Design review of the part shown in the three views and the two pictorial views. Dimensions are in mm from the part's minimum x, y and z. A direction names the side the tool comes from. Round coordinates to 2 decimals unless told otherwise and drop trailing zeros. Write each loop counter-clockwise with the first axis right and the second up, starting at its lowest first coordinate (ties: lowest second). Pieces come first, ordered by that corner, then holes. Notation, with made-up numbers: (-16, 36.25) -> (28, 36.25) arc R18 ccw to (28, 47.25) -> close; hole circle Ø5 at (88.5, 50.25). An arc over 180 degrees is marked (long way). One line per question, with ' | ' between items. Start each with the question number.
1) Insertion check: pin 1 Ø0.8 at (x, y) = (8.5, 15) entering from -Z; pin 2 Ø1.5 at (y, z) = (12, 33.5) entering from +X; pin 3 Ø1.1 at (y, z) = (15.5, 14.5) entering from +X. Each pin has a flat end and moves straight along its axis. Give the tip position at first contact, or say it passes through.
2) Consider section C-C (z = 9). Give the boundary of the cut face in (x, y).
3) Consider section A-A (y = 5). Give the boundary of the cut face in (x, z), then the cut area to 4 significant figures.
4) For the marked faces 1 and 2, list the 3-axis set-ups (+Z, -Z, +X, -X, +Y, -Y) from which the entire face can be reached by the end or side of a thin tool; tool diameter is ignored.
5) Consider section B-B (z = 46). Give the boundary of the cut face in (x, y).
6) For probe 1 along Y at (x, z) = (9, 35.5); probe 2 along Z at (x, y) = (13.25, 15), list the stretches that pass through material, from the lowest coordinate up.
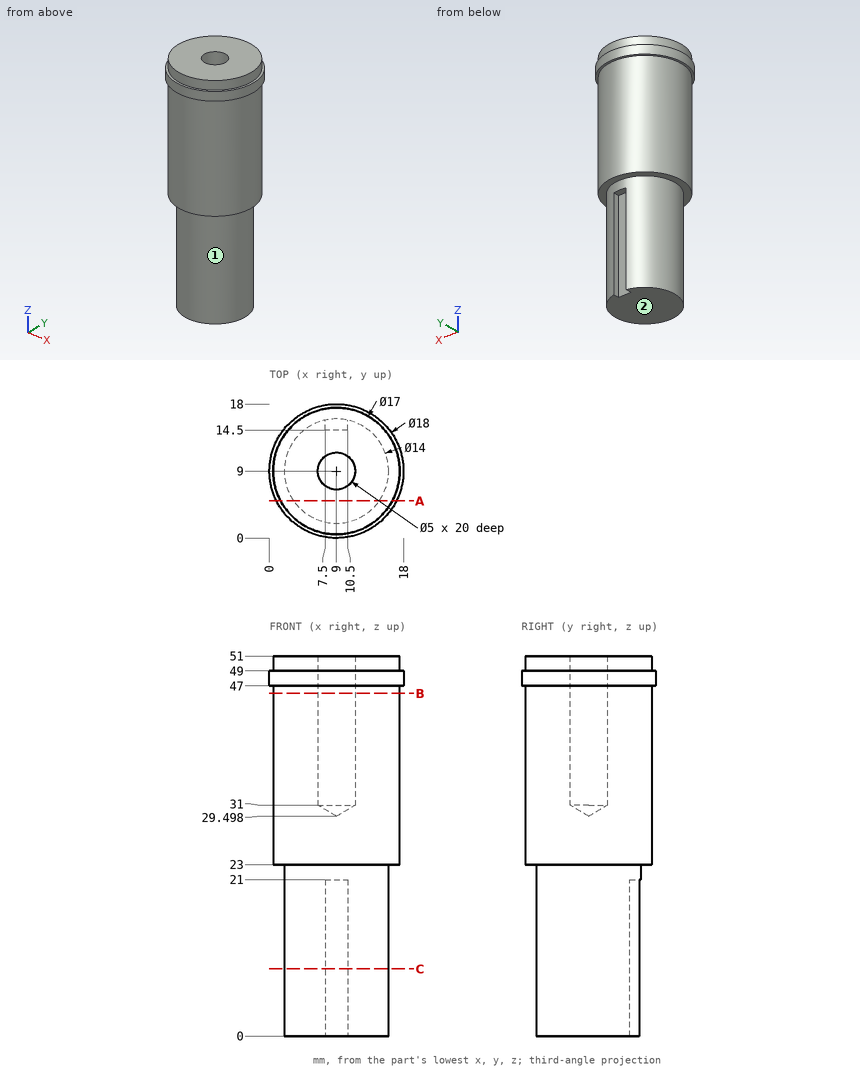
From the geometry:
1) pin 1: stops at z = 21 | pin 2: stops at x = 17.2 | pin 3: stops at x = 12.69
2) outline: (7.5, 14.5) -> (7.5, 15.84) arc R7 ccw (long way) to (10.5, 15.84) -> (10.5, 14.5) -> close
3) outline: (0.94, 47) -> (1.5, 47) -> (1.5, 23) -> (3.26, 23) -> (3.26, 0) -> (14.74, 0) -> (14.74, 23) -> (16.5, 23) -> (16.5, 47) -> (17.06, 47) -> (17.06, 49) -> (16.5, 49) -> (16.5, 51) -> (1.5, 51) -> (1.5, 49) -> (0.94, 49) -> close | area: 686.5 mm2
4) face 1: -Z | face 2: -Z, +X, -X, +Y, -Y
5) outline: circle Ø17 at (9, 9); hole circle Ø5 at (9, 9)
6) probe 1: y = 0.5 to 6.5, 11.5 to 17.5 | probe 2: z = 23 to 51
